Check sheet for the modelled part. Datum: model origin and axes. Units: mm. A direction names the side the tool comes from. Give positions to 0.01 mm unless a question says otherwise; leave off trailing zeros. Write each loop counter-clockwise with the first axis right and the second up, starting at its lowest first coordinate (ties: lowest second). Pieces come first, ordered by that corner, then holes. Notation, with made-up numbers: M 88,-9 L 138,-9 A34 cw 138,29 Z; hole C 18,40 d2. An arc over 180 degrees is marked long. Write item = value, one per line. Start each with the question number.
1) Cross-section at C-C, the plane y = 19. Record the cut outline in (x, z), plus the area to 3 significant figures.
2) Cross-section at A-A, the plane z = 21.5. Record the cut outline in (x, y).
3) Cross-section at B-B, the plane x = -2. Record the cut outline in (y, z), plus the area to 3 significant figures.
4) Access from +Z, -Z, +X, -X, +Y, -Y to the whole of each face (thin tool, end or side, straight path). Record for faces 1 (the flat face through (51, 6, 0)), 2 (the flat face through (-54, 3, 0)), 3 (the flat face through (11, 24, -33)), 4 (the flat face through (-46, 6, 0)), 5 (the flat face through (53.93, 28.365, 8.293)).
5) Scan lines: line 1 along Z through (x, y) = (36, 40.5); line 2 along X through (y, z) = (42.5, 5.5); line 3 along X through (y, z) = (4.05, 18.8). Record each from-to range of solid material in increasing order. Write a range as [from, to].
6) Mould release check, pull along Y, two halves, no side actions. Record for faces 6 (the flat face through (53.93, 37.635, -8.293)), 7 (the flat face through (59, 3, 21)), 8 (the flat face through (53.93, 28.135, -8.16)), 9 (the cylindrical face through (12.67, 34.69, 42.86)): released by +Y, released by -Y, zero draft, split by the parting line, or undercut.
7) Cross-section at D-D, the plane z = 41. Record the cut outline in (x, y).
8) Go/stop test with flat-tipped pins: pin 1 (9.5 mm diameter, centred on y = 32.5, z = 3, fed in from +X); pin 2 (20 mm diameter, centred on x = 1.5, y = 40.5, fed in from +Z); pin 3 (12 mm diameter, centred on y = 47, z = -12.5, fed in from +X); pin 4 (25 mm diameter, centred on x = 11.5, y = 18, fed in from +Z). Record where each tip stops, or that it passes through.
```python
from build123d import *

# Parameters (mm, degrees)
SZKIC1_R                    = 4.5
DODANIE_WYCI_GNI_CIE1_DEPTH = 6
SZKIC2_W                    = 87
SZKIC2_H                    = 52
DODANIE_WYCI_GNI_CIE2_DEPTH = 60
SZKIC3_R                    = 25
DODANIE_WYCI_GNI_CIE3_DEPTH = 7
SZKIC4_R                    = 6.75
DODANIE_WYCI_GNI_CIE4_DEPTH = 20
DODANIE_WYCI_GNI_CIE5_DEPTH = 10


with BuildPart() as part:
    # Szkic1 → Dodanie-wyciągnięcie1 (new body)
    with BuildSketch(Plane(origin=(0, 0, 0), x_dir=(1, 0, 0), z_dir=(0, 1, 0))):
        with BuildLine():
            Line((64, 16), (54, 26))
            Line((54, 26), (-54, 26))
            Line((-54, 26), (-54, -26))
            Line((-54, -26), (54, -26))
            Line((54, -26), (64, -16))
            Line((64, -16), (64, -4.25))
            Line((64, -4.25), (56.25, -4.25))
            ThreePointArc((56.25, -4.25), (52, 0), (56.25, 4.25))
            Line((56.25, 4.25), (64, 4.25))
            Line((64, 4.25), (64, 16))
        make_face()
        with Locations(Location((-46, -18.8, 0), (0, 0, 270))):
            Circle(SZKIC1_R, mode=Mode.SUBTRACT)
        with Locations(Location((-46, 18.8, 0), (0, 0, 270))):
            Circle(SZKIC1_R, mode=Mode.SUBTRACT)
    extrude(amount=DODANIE_WYCI_GNI_CIE1_DEPTH)

    # Szkic2 → Dodanie-wyciągnięcie2 (add)
    with BuildSketch(Plane(origin=(0, 6, 0), x_dir=(1, 0, 0), z_dir=(0, 1, 0))):
        with Locations((5.5, 0)):
            Rectangle(SZKIC2_W, SZKIC2_H)
    extrude(amount=DODANIE_WYCI_GNI_CIE2_DEPTH)

    # Szkic3 → Dodanie-wyciągnięcie3 (add)
    with BuildSketch(Plane(origin=(0, 0, -26), x_dir=(-1, 0, 0), z_dir=(0, 0, -1))):
        with Locations((-16.3, 29)):
            Circle(SZKIC3_R)
    dodanie_wyci_gni_cie3 = extrude(amount=DODANIE_WYCI_GNI_CIE3_DEPTH)

    # Szkic4 → Dodanie-wyciągnięcie4 (add)
    with BuildSketch(Plane(origin=(0, 0, -33), x_dir=(-1, 0, 0), z_dir=(0, 0, -1))):
        with Locations((-16.3, 29)):
            Circle(SZKIC4_R)
    dodanie_wyci_gni_cie4 = extrude(amount=DODANIE_WYCI_GNI_CIE4_DEPTH)

    # Lustro1: Dodanie-wyciągnięcie3, Dodanie-wyciągnięcie4 across plane
    add(dodanie_wyci_gni_cie3.mirror(Plane.XY))
    add(dodanie_wyci_gni_cie4.mirror(Plane.XY))

    # Szkic5 → Dodanie-wyciągnięcie5 (add)
    with BuildSketch(Plane(origin=(49, 0, 0), x_dir=(0, 0, -1), z_dir=(1, 0, 0))):
        Polygon((5.428883431, 23.467919533), (10.969465551, 32.935510732), (5.54058212, 42.467591199), (-5.428883431, 42.532080467), (-10.969465551, 33.064489268), (-5.54058212, 23.532408801), align=None)
    extrude(amount=DODANIE_WYCI_GNI_CIE5_DEPTH)


solid = part.part
```
Reply:
q1.outline = M -38,-26 L -6.61,-26 L -6.61,-33 L 39.21,-33 L 39.21,-26 L 49,-26 L 49,26 L 39.21,26 L 39.21,33 L -6.61,33 L -6.61,26 L -38,26 Z
q1.area = 5,170 mm2
q2.outline = M -54,0 L -49.6,0 L -49.6,6 L -54,6 Z; M -42.4,0 L 58.5,0 L 58.5,6 L 49,6 L 49,66 L -38,66 L -38,6 L -42.4,6 Z
q3.outline = M 0,-26 L 11.97,-26 L 11.97,-33 L 46.03,-33 L 46.03,-26 L 66,-26 L 66,26 L 46.03,26 L 46.03,33 L 11.97,33 L 11.97,26 L 0,26 Z
q3.area = 3,910 mm2
q4.face_1 = +Z, -Z, +X
q4.face_2 = +Z, -Z, -X, +Y, -Y
q4.face_3 = -Z
q4.face_4 = +Z, -Z, -X, +Y
q4.face_5 = +Z, +X
q5.line_1 = [-33, 33]
q5.line_2 = [-38, 49]
q5.line_3 = [-54, -50.5], [-41.5, 61.2]
q6.face_6 = released by +Y
q6.face_7 = zero draft
q6.face_8 = undercut
q6.face_9 = split by the parting line
q7.outline = C 16.3,29 d13.5
q8.pin_1 = 59
q8.pin_2 = 33
q8.pin_3 = 49
q8.pin_4 = 53
